```python
from build123d import *

# Parameters (mm, degrees)
EXTRUDE_THIN1_DEPTH       = 76.2
SKETCH2_R                 = 3.175
BOSS_EXTRUDE1_DEPTH       = 3.175
LPATTERN1_COUNT           = 3
LPATTERN1_PITCH           = 30.1625
LPATTERN1_COPY_1_SKETCH_R = 3.175
LPATTERN1_COPY_1_DEPTH    = 3.175
LPATTERN1_COPY_2_SKETCH_R = 3.175
LPATTERN1_COPY_2_DEPTH    = 3.175


with BuildPart() as part:
    # Sketch1 → Extrude-Thin1 (new body)
    with BuildSketch(Plane.XY):
        with BuildLine():
            Line((92.701547158, 0), (86.929349905, 0))
            ThreePointArc((86.929349905, 0), (86.386392927, 0.095737965), (85.908924574, 0.371404447))
            Line((85.908924574, 0.371404447), (74.641391347, 9.825987422))
            ThreePointArc((74.641391347, 9.825987422), (74.163922994, 10.101653904), (73.620966016, 10.197391869))
            Line((73.620966016, 10.197391869), (11.27657151, 10.197391869))
            ThreePointArc((11.27657151, 10.197391869), (10.733614533, 10.101653904), (10.25614618, 9.825987422))
            Line((10.25614618, 9.825987422), (-1.011387048, 0.371404447))
            ThreePointArc((-1.011387048, 0.371404447), (-1.488855401, 0.095737965), (-2.031812378, 0))
            Line((-2.031812378, 0), (-7.804009631, 0))
            Line((-7.804009631, 0), (-7.804009631, -2.032))
            Line((-7.804009631, -2.032), (-2.031812378, -2.032))
            ThreePointArc((-2.031812378, -2.032), (-0.793870469, -1.813717441), (0.294757375, -1.185197862))
            Line((0.294757375, -1.185197862), (11.438356279, 8.165391869))
            Line((11.438356279, 8.165391869), (73.459181247, 8.165391869))
            Line((73.459181247, 8.165391869), (84.602780151, -1.185197862))
            ThreePointArc((84.602780151, -1.185197862), (85.691407996, -1.813717441), (86.929349905, -2.032))
            Line((86.929349905, -2.032), (92.701547158, -2.032))
            Line((92.701547158, -2.032), (92.701547158, 0))
        make_face()
    extrude(amount=-EXTRUDE_THIN1_DEPTH)

    # Sketch2 → Boss-Extrude1 (add)
    with BuildSketch(Plane(origin=(0, 0, 0), x_dir=(1, 0, 0), z_dir=(0, 1, 0))):
        with BuildLine():
            Line((94.289047158, 1.5875), (102.226547158, 1.5875))
            ThreePointArc((102.226547158, 1.5875), (108.576547158, 7.9375), (102.226547158, 14.2875))
            Line((102.226547158, 14.2875), (94.289047158, 14.2875))
            ThreePointArc((94.289047158, 14.2875), (93.166515143, 14.752467985), (92.701547158, 15.875))
            Line((92.701547158, 15.875), (92.701547158, 0))
            ThreePointArc((92.701547158, 0), (93.166515143, 1.122532015), (94.289047158, 1.5875))
        make_face()
        with Locations(Location((102.226547158, 7.9375, 0), (0, 0, 270))):
            Circle(SKETCH2_R, mode=Mode.SUBTRACT)
    boss_extrude1 = extrude(amount=-BOSS_EXTRUDE1_DEPTH)

    # Mirror1: Boss-Extrude1 across plane
    add(boss_extrude1.mirror(Plane(origin=(42.448768763, 0, 0), x_dir=(0, 0, 1), z_dir=(1, 0, 0))))

    # LPattern1: Boss-Extrude1 ×3
    with Locations(*[(0, 0, -i * LPATTERN1_PITCH) for i in range(1, LPATTERN1_COUNT)]):
        add(boss_extrude1)

    # LPattern1 copy 1 sketch → LPattern1 copy 1 (add)
    with BuildSketch(Plane(origin=(84.897537526, 0, -30.1625), x_dir=(-1, 0, 0), z_dir=(0, 1, 0))):
        with BuildLine():
            Line((94.289047158, -1.5875), (102.226547158, -1.5875))
            ThreePointArc((102.226547158, -1.5875), (108.576547158, -7.9375), (102.226547158, -14.2875))
            Line((102.226547158, -14.2875), (94.289047158, -14.2875))
            ThreePointArc((94.289047158, -14.2875), (93.166515143, -14.752467985), (92.701547158, -15.875))
            Line((92.701547158, -15.875), (92.701547158, 0))
            ThreePointArc((92.701547158, 0), (93.166515143, -1.122532015), (94.289047158, -1.5875))
        make_face()
        with Locations((102.226547158, -7.9375)):
            Circle(LPATTERN1_COPY_1_SKETCH_R, mode=Mode.SUBTRACT)
    extrude(amount=-LPATTERN1_COPY_1_DEPTH)

    # LPattern1 copy 2 sketch → LPattern1 copy 2 (add)
    with BuildSketch(Plane(origin=(84.897537526, 0, -60.325), x_dir=(-1, 0, 0), z_dir=(0, 1, 0))):
        with BuildLine():
            Line((94.289047158, -1.5875), (102.226547158, -1.5875))
            ThreePointArc((102.226547158, -1.5875), (108.576547158, -7.9375), (102.226547158, -14.2875))
            Line((102.226547158, -14.2875), (94.289047158, -14.2875))
            ThreePointArc((94.289047158, -14.2875), (93.166515143, -14.752467985), (92.701547158, -15.875))
            Line((92.701547158, -15.875), (92.701547158, 0))
            ThreePointArc((92.701547158, 0), (93.166515143, -1.122532015), (94.289047158, -1.5875))
        make_face()
        with Locations((102.226547158, -7.9375)):
            Circle(LPATTERN1_COPY_2_SKETCH_R, mode=Mode.SUBTRACT)
    extrude(amount=-LPATTERN1_COPY_2_DEPTH)


solid = part.part
```
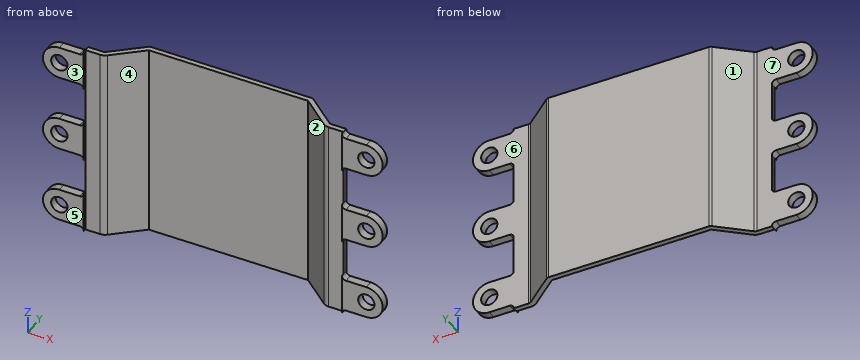
Work out the finished part from the listing and answer in its coordinate system (mm). Face numbers are marked on the shaded views. A direction names the side the tool comes from. Round coordinates to 2 decimals unless told otherwise and drop trailing zeros. Order: outer loops, then holes, each group sorted by start corner. A loop starts at its lowest first (then second) coordinate and runs counter-clockwise, first axis right, second up.
Q1. The mould has two halves that part along X. Classify the marked faces 1, 2 and 3: pulls with the +X half, pulls with the -X half, needs draft (parallel to the pull), parting line crosses it, or undercut.
Solution:
face 1: pulls with the -X half
face 2: undercut
face 3: needs draft
Q2. Find the intervals of material crossed by line 1 along Y through (x, z) = (42, -6); line 2 along X through (y, z) = (4.5, -11); line 3 along X through (y, z) = (1.5, -25), in increasing order.
Solution:
line 1: y = 8.17 to 10.2
line 2: x = 3.91 to 7.07, 77.83 to 80.99
line 3: x = 0.33 to 3.49, 81.4 to 84.56
Q3. A tool of negligible diameter and unlimited length cuts with its end or side. For the marked faces 4, 5, 6 and 7, from which of +Z, -Z, +X, -X, +Y, -Y can it reach the whole face along a straight path? Write none if from no direction.
Solution:
face 4: +Z, -Z, -Y
face 5: +Z, -Z, +X, -X, -Y
face 6: +Z, -Z, +X, +Y
face 7: +Z, -Z, -X, +Y
Q4. A cutting plane is placed at C-C, the plane y = 5.75. Determine the outline of the cut face in (x, z).
Solution:
outline: (5.4, -76.2) - (8.56, -76.2) - (8.56, 0) - (5.4, 0) - close; (76.34, -76.2) - (79.5, -76.2) - (79.5, 0) - (76.34, 0) - close
Q5. A cutting plane is placed at A-A, the plane x = -11.5. Count the separate pieces of the cut face and the enclosed holes in it, then the cut area to 3 significant figures.
Solution:
separate pieces: 3
enclosed holes: 0
area: 121 mm2
Q6. Given pin 1 Ø1.5 at (y, z) = (1, -13.5) entering from +X; pin 2 Ø1 at (x, y) = (-12, -1) entering from +Z; pin 3 Ø1 at (y, z) = (-1, -22) entering from -X; pin 4 Ø4 at (x, z) = (-17.33, -38.1) entering from +Y, each flat-ended and moving along its own axis, determine where each tip first touches the part or whether it passes through.
Solution:
pin 1: stops at x = 86.07
pin 2: stops at z = -1.59
pin 3: stops at x = -7.8
pin 4: passes through
